Geometry: final body of the model. Coordinates: model frame, mm. A direction names the side the tool comes from. Give positions to 0.01 mm unless a question says otherwise; leave off trailing zeros. Loops run counter-clockwise (first coordinate to the right, second up) from the corner with the lowest first, then second, coordinate; pieces in that order, holes last. Notation, with made-up numbers: (4.25, 9.25) -> (29.25, 9.25) arc R25 cw to (29.25, 34.25) -> close; hole circle Ø1 at (51.5, 85.5). An arc over 180 degrees is marked (long way). Answer in a Markdown table with one row per item. Add a question column.
1) Draft query along Z for faces 1 (the flat face through (31, -18.918, -39)), 2 (the flat face through (30, -2.54, -20)), 3 (the flat face through (30, -7, -39.872)), 4 (the flat face through (30.2, -8.7, -37.332)). Return one class per face: +Z half, -Z half, draft (parallel to the pull), parting line (faces both ways), or undercut.
2) Section query D-D (y = -12.25). Return the cut outline in (x, z).
3) Section query C-C (z = -14). Return the cut outline in (x, y).
4) Section query B-B (x = 30.5). Return the cut outline in (y, z).
5) Access query for faces 5 (the flat face through (2.54, -14, -20)), 6 (the flat face through (61.249, -13, -20)), 7 (the flat face through (26.084, -14, -39)). Directions: +Z, -Z, +X, -X, +Y, -Y. A direction counts if a zero-diameter tool reaches every point of the face in a straight line with its end or side. Return the directions, or none.
6) Line query: line 1 (X direction, y = -14.75, z = -21); line 2 (Z direction, x = 3, y = -13); line 3 (Y direction, x = 16.5, z = -7). Output: solid intervals per line, ascending. Write a range as from..to.
7) First-contact query: P1, Ø0.8, axis at x = 30.5, z = -38.5, coming from the +Y side; P2, Ø1, axis at x = 54.5, z = -22.5, coming from the -Y side. Flat tips, straight axial feed; report the tip coordinate or a pass-through.
8) Section query A-A (y = -20.75). Return the cut outline in (x, z), plus the area to 3 significant figures.
```python
from build123d import *

# Parameters (mm, degrees)
F0_W     = 61.248694
F0_H     = 39.8717
F1_DEPTH = 25.4
F2_T     = -2.54
F3_W     = 9.080695
F3_H     = 9.89195
F4_DEPTH = 25.4


with BuildPart() as f1:
    # F0 (on Front) → F1 (new body)
    with BuildSketch(Plane.XZ):
        with Locations((30.624347, -19.93585)):
            Rectangle(F0_W, F0_H)
    extrude(amount=F1_DEPTH)

    # F2
    f2_openings = [f1.faces().sort_by_distance(p)[0] for p in [
        (30.624347, -25.4, -19.93585),
    ]]
    offset(amount=F2_T, openings=f2_openings)

    # F3 (on face) → F4 (cut)
    with BuildSketch(Plane(origin=(0, 0, -39.8717), x_dir=(1, 0, 0), z_dir=(0, 0, -1))):
        with Locations((30.624346, 13.972152)):
            Rectangle(F3_W, F3_H)
    extrude(amount=-F4_DEPTH, mode=Mode.SUBTRACT)


solid = f1.part
```
Evaluation:
| question | item | result |
|---|---|---|
| 1 | face 1 | draft |
| 1 | face 2 | undercut |
| 1 | face 3 | -Z half |
| 1 | face 4 | undercut |
| 2 | outline | (0, -39.87) -> (26.08, -39.87) -> (26.08, -37.33) -> (2.54, -37.33) -> (2.54, -2.54) -> (58.71, -2.54) -> (58.71, -37.33) -> (35.16, -37.33) -> (35.16, -39.87) -> (61.25, -39.87) -> (61.25, 0) -> (0, 0) -> close |
| 3 | outline | (0, -25.4) -> (2.54, -25.4) -> (2.54, -2.54) -> (58.71, -2.54) -> (58.71, -25.4) -> (61.25, -25.4) -> (61.25, 0) -> (0, 0) -> close |
| 4 | outline | (-25.4, -39.87) -> (-18.92, -39.87) -> (-18.92, -37.33) -> (-25.4, -37.33) -> close; (-25.4, -2.54) -> (-2.54, -2.54) -> (-2.54, -37.33) -> (-9.03, -37.33) -> (-9.03, -39.87) -> (0, -39.87) -> (0, 0) -> (-25.4, 0) -> close |
| 5 | face 5 | -Y |
| 5 | face 6 | +Z, -Z, +X, +Y, -Y |
| 5 | face 7 | -Z |
| 6 | line 1 | 0..2.54, 58.71..61.25 |
| 6 | line 2 | -39.87..-37.33, -2.54..0 |
| 6 | line 3 | -2.54..0 |
| 7 | P1 | y = 0 |
| 7 | P2 | y = -2.54 |
| 8 | outline | (0, -39.87) -> (61.25, -39.87) -> (61.25, 0) -> (0, 0) -> close; hole (2.54, -37.33) -> (58.71, -37.33) -> (58.71, -2.54) -> (2.54, -2.54) -> close |
| 8 | area | 488 mm² |
